For this review, take the finished solid that the model builds, in its own axes (mm). A direction names the side the tool comes from. Give positions to 0.01 mm unless a question says otherwise; leave off trailing zeros. Write each loop counter-clockwise with the first axis right and the second up, starting at its lowest first coordinate (ties: lowest second). Pieces come first, ordered by that corner, then holes. Notation, with made-up numbers: M 36,9 L 54,9 A14 cw 54,15 Z; hole C -36,-33.5 d3. An arc over 180 degrees is marked long. Use one line per item in the form item = value. Start each with the question number.
Q1. Consider section C-C on z = 917.5. Write out the cut boundary in (x, y), and give its area (3 significant figures).
Q2. Consider section B-B on x = 469.5. Write out the cut boundary in (y, z), and give its area (3 significant figures).
Q3. Tool access review of faces 1 (the cylindrical face through (501.805, -19.014, 1537.627)), 2 (the flat face through (560, -119, 381.881)), 3 (the flat face through (560, -119, 361.881)): name each direction out of +Z, -Z, +X, -X, +Y, -Y from which nothing blocks a thin tool from reaching the whole face with its end or side.
Q4. Clearance check with flat-ended pins moving along their axes: pin 1 Ø22 at (y, z) = (-120, 369.5) entering from +X; pin 2 Ø4 at (x, y) = (356.5, -91.5) entering from -Z; pin 3 Ø6 at (x, z) = (283, 995) entering from -Y. State where each tip first meets the part, or that it passes through.
Q5. Mouldability with a two-part tool opening along X and no side actions: class faces 4 (the flat face through (574, -119, 211.881)), 5 (the flat face through (560, -18, 1049)) as released by +X, released by -X, zero draft, split by the parting line, or undercut.
Q6. For probe 1 along Z at (x, y) = (987, -40.5); probe 2 along Y at (x, z) = (1013, 719.5); probe 3 along Y at (x, z) = (725.5, 765), list the stretches that pass through material, from the lowest coordinate up. Write a range as [from, to].
Q7. Consider section D-D on z = 1190. Write out the cut boundary in (x, y).
Q8. Consider section A-A on y = -104.5. Write out the cut boundary in (x, z), and give its area (3 significant figures).
```python
from build123d import *

# Parameters (mm, degrees)
F0_W     = 1200
F0_H     = 1700
F1_DEPTH = 20
F2_R     = 500
F3_DEPTH = 2
F4_W     = 1000
F4_H     = 20
F5_DEPTH = 200


with BuildPart() as f1:
    # F0 (on Front) → F1 (new body)
    with BuildSketch(Plane.XZ):
        with Locations((566.895331, 791.881418)):
            Rectangle(F0_W, F0_H)
    extrude(amount=F1_DEPTH)

    # F2 (on face) → F3 (cut)
    with BuildSketch(Plane.XZ.offset(20)):
        with Locations((566.895331, 1041.881418)):
            Circle(F2_R)
    extrude(amount=-F3_DEPTH, mode=Mode.SUBTRACT)

    # F4 (on face) → F5 (join)
    with BuildSketch(Plane.XZ.offset(20)):
        Polygon((66.895331, 191.881418), (566.895331, 191.881418), (1066.895331, 191.881418), (1066.895331, 211.881418), (66.895331, 211.881418), align=None)
        with Locations((566.895331, 371.881418)):
            Rectangle(F4_W, F4_H)
    extrude(amount=F5_DEPTH)


solid = f1.part
```
Working result:
q1.outline = M -33.1,-20 L 82.61,-20 L 82.61,-18 L 1051.18,-18 L 1051.18,-20 L 1166.9,-20 L 1166.9,0 L -33.1,0 Z
q1.area = 22,100 mm²
q2.outline = M -220,191.88 L -20,191.88 L -20,-58.12 L 0,-58.12 L 0,1641.88 L -20,1641.88 L -20,1532.3 L -18,1532.3 L -18,551.46 L -20,551.46 L -20,381.88 L -220,381.88 L -220,361.88 L -20,361.88 L -20,211.88 L -220,211.88 Z
q2.area = 40,000 mm²
q3.face_1 = -Y
q3.face_2 = +Z, +X, -X, -Y
q3.face_3 = +X, -X, -Y
q4.pin_1 = 1066.9
q4.pin_2 = 191.88
q4.pin_3 = -18
q5.face_4 = zero draft
q5.face_5 = undercut
q6.probe_1 = [191.88, 211.88], [361.88, 381.88]
q6.probe_2 = [-20, 0]
q6.probe_3 = [-18, 0]
q7.outline = M -33.1,-20 L 89.34,-20 L 89.34,-18 L 1044.45,-18 L 1044.45,-20 L 1166.9,-20 L 1166.9,0 L -33.1,0 Z
q8.outline = M 66.9,191.88 L 1066.9,191.88 L 1066.9,211.88 L 66.9,211.88 Z; M 66.9,361.88 L 1066.9,361.88 L 1066.9,381.88 L 66.9,381.88 Z
q8.area = 40,000 mm²
